Read the model definition and answer for the solid it produces. Units are mm, in the model's axes. A direction names the side the tool comes from. Coordinates: 2 decimals unless noted, no trailing zeros. Order: outer loops, then holes, each group sorted by start corner. A loop starts at its lowest first (then second) coordinate and runs counter-clockwise, first axis right, second up. Notation, with made-up numbers: (62.25, 38.25) -> (75.25, 38.25) arc R10 ccw to (75.25, 46.25) -> close; hole circle Ø10 at (-9, 27.25). An arc over 180 degrees is marked (long way). Answer as a JSON object with one key per item and string values. Group by question number.
1) A tool of negligible diameter and unlimited length cuts with its end or side. For faces 5 (the flat face through (5, 0, 0)), 6 (the flat face through (2, 3.528, 3)), from which of +Z, -Z, +X, -X, +Y, -Y can it reach the whole face along a straight path? Write none if from no direction.
2) Section C-C on z = 0.5 is taken. Determine the outline of the cut face in (x, y), and give its area (3 significant figures).
3) Determine the mould class of faces 1 (the flat face through (2, -3.472, -3)), 2 (the flat face through (2, 6.528, 0)), 3 (the flat face through (2.46, -3.08, -0.41)), 4 (the cylindrical face through (2.465, 0.171, 12.995)) for opening direction Y: released by +Y, released by -Y, zero draft, split by the parting line, or undercut.
4) Section A-A on x = 2.3 is taken. Count the separate pieces of the cut face and the enclosed holes in it, and give its area (3 significant figures).
5) Consider L1, parallel to Y at x = 3.4, z = -2; L2, parallel to Z at x = 2.55, y = -1.75; L3, parallel to Y at x = 1.15, z = -4.25. Determine where each line is inside the solid, lowest interval first.
6) Section B-B on z = 10.75 is taken. Determine the outline of the cut face in (x, y), and give its area (3 significant figures).
7) Given pin 1 (2.5 mm diameter, centred on y = 0.03, z = 4.75, fed in from -X); pin 2 (1.1 mm diameter, centred on x = 1.5, y = -1.5, fed in from -Z); pin 3 (1 mm diameter, centred on x = 3, y = 1, fed in from +Z); pin 4 (1 mm diameter, centred on x = 4, y = -4, fed in from +Z), each flat-ended and moving along its own axis, determine where each tip first touches the part or whether it passes through.
from build123d import *

# Parameters (mm, degrees)
SKETCH2_R           = 1.7
BOSS_EXTRUDE2_DEPTH = 5
CHAMFER1_SIZE       = 1.8


with BuildPart() as part:
    # Sketch2 → Boss-Extrude2 (new body)
    with BuildSketch(Plane.YZ):
        with BuildLine():
            Line((-6.472145094, 6.496243265), (-6.472145094, -6.503756735))
            ThreePointArc((-6.472145094, -6.503756735), (0.027854906, -13.003756735), (6.527854906, -6.503756735))
            Line((6.527854906, -6.503756735), (6.527854906, 6.496243265))
            ThreePointArc((6.527854906, 6.496243265), (0.027854906, 12.996243265), (-6.472145094, 6.496243265))
        make_face()
        with Locations(Location((0.027854906, 4.746243265, 0), (0, 0, 270))):
            Circle(SKETCH2_R, mode=Mode.SUBTRACT)
        with Locations(Location((0.027854906, -4.753756735, 0), (0, 0, 270))):
            Circle(SKETCH2_R, mode=Mode.SUBTRACT)
        with BuildLine():
            Line((-5.272145094, 6.496243265), (-5.272145094, -6.503756735))
            ThreePointArc((-5.272145094, -6.503756735), (-5.076205272, -7.931541625), (-4.502873512, -9.253756735))
            Line((-4.502873512, -9.253756735), (0.027854906, -9.253756735))
            ThreePointArc((0.027854906, -9.253756735), (2.673606218, -8.045044583), (3.491956522, -5.253756735))
            ThreePointArc((3.491956522, -5.253756735), (-0.222788612, -8.244770603), (-3.472145094, -4.753756735))
            Line((-3.472145094, -4.753756735), (-3.472145094, -0.803756735))
            Line((-3.472145094, -0.803756735), (-2.672145094, -0.003756735))
            Line((-2.672145094, -0.003756735), (-3.472145094, 0.796243265))
            Line((-3.472145094, 0.796243265), (-3.472145094, 2.609365837))
            ThreePointArc((-3.472145094, 2.609365837), (-4.263608941, 7.662838695), (0.027854906, 10.446243265))
            Line((0.027854906, 10.446243265), (3.561620603, 10.446243265))
            ThreePointArc((3.561620603, 10.446243265), (-2.135596249, 11.334577596), (-5.272145094, 6.496243265))
        make_face(mode=Mode.SUBTRACT)
        with BuildLine():
            Line((4.558583325, 9.246243265), (0.027854906, 9.246243265))
            ThreePointArc((0.027854906, 9.246243265), (-2.617896405, 8.037531112), (-3.436246709, 5.246243265))
            ThreePointArc((-3.436246709, 5.246243265), (0.278498425, 8.237257133), (3.527854906, 4.746243265))
            Line((3.527854906, 4.746243265), (3.527854906, 0.796243265))
            Line((3.527854906, 0.796243265), (2.727854906, -0.003756735))
            Line((2.727854906, -0.003756735), (3.527854906, -0.803756735))
            Line((3.527854906, -0.803756735), (3.527854906, -2.616879307))
            ThreePointArc((3.527854906, -2.616879307), (4.319318754, -7.670352166), (0.027854906, -10.453756735))
            Line((0.027854906, -10.453756735), (-3.50591079, -10.453756735))
            ThreePointArc((-3.50591079, -10.453756735), (2.191306062, -11.342091066), (5.327854906, -6.503756735))
            Line((5.327854906, -6.503756735), (5.327854906, 6.496243265))
            ThreePointArc((5.327854906, 6.496243265), (5.131915085, 7.924028155), (4.558583325, 9.246243265))
        make_face(mode=Mode.SUBTRACT)
    extrude(amount=BOSS_EXTRUDE2_DEPTH)

    # Chamfer1
    chamfer1_edges = [part.edges().sort_by_distance(p)[0] for p in [
        (5, 0.027854906, 6.446243265),
        (5, 0.027854906, -3.053756735),
    ]]
    chamfer(chamfer1_edges, length=CHAMFER1_SIZE - 0.0001)  # a hair under: the kernel refuses the full size


solid = part.part
Worked answers:
{
 "1": {"face 5": "+Z, -Z, +X, +Y, -Y", "face 6": "+X, -X"},
 "2": {"outline": "(0, -6.47) -> (5, -6.47) -> (5, -5.27) -> (0, -5.27) -> close; (0, -3.18) -> (5, -3.18) -> (5, 3.23) -> (0, 3.23) -> close; (0, 5.33) -> (5, 5.33) -> (5, 6.53) -> (0, 6.53) -> close", "area": "44.0 mm²"},
 "3": {"face 1": "undercut", "face 2": "released by +Y", "face 3": "undercut", "face 4": "split by the parting line"},
 "4": {"separate pieces": "1", "enclosed holes": "4", "area": "192 mm²"},
 "5": {"L1": "y = -6.47 to -5.27, -3.47 to 3.53, 5.33 to 6.53", "L2": "z = -12.76 to -11.5, -10.45 to -9.25, -7.77 to 7.76, 8.76 to 10.1, 11.49 to 12.75", "L3": "y = -6.47 to -5.27, -3.47 to -1.6, 1.65 to 4.48, 5.33 to 6.53"},
 "6": {"outline": "(0, -4.89) -> (5, -4.89) -> (5, -3.13) -> (0, -3.13) -> close; (0, 3.19) -> (5, 3.19) -> (5, 4.94) -> (0, 4.94) -> close", "area": "17.5 mm²"},
 "7": {"pin 1": "passes through", "pin 2": "stops at z = -12.93", "pin 3": "stops at z = 12.98", "pin 4": "stops at z = 11.96"}
}
